from build123d import *

# Parameters (mm, degrees)
SKETCH1_W                      = 124
SKETCH1_H                      = 219.6
SKETCH1_R                      = 3.5
BOSS_EXTRUDE1_DEPTH            = 3.125
SKETCH2_R                      = 2.5
CUT_EXTRUDE1_DEPTH             = 10
M5_CLEARANCE_HOLE1_D           = 5.5
M5_CLEARANCE_HOLE1_DEPTH       = 10.1
M5_CLEARANCE_HOLE1_CSINK_D     = 5.55
M5_CLEARANCE_HOLE1_CSINK_ANGLE = 90
M5_CLEARANCE_HOLE1_TIP         = 1.652366702
M5_CLEARANCE_HOLE2_D           = 5.5
M5_CLEARANCE_HOLE2_DEPTH       = 10.1
M5_CLEARANCE_HOLE2_CSINK_D     = 5.55
M5_CLEARANCE_HOLE2_CSINK_ANGLE = 90
M5_CLEARANCE_HOLE2_TIP         = 1.652366702
M5_CLEARANCE_HOLE3_D           = 5.5
M5_CLEARANCE_HOLE3_CSINK_D     = 5.55
M5_CLEARANCE_HOLE3_CSINK_ANGLE = 90


with BuildPart() as part:
    # Sketch1 → Boss-Extrude1 (new body)
    with BuildSketch(Plane(origin=(0, 0, 0), x_dir=(1, 0, 0), z_dir=(0, 1, 0))):
        with Locations((62, 109.8)):
            Rectangle(SKETCH1_W, SKETCH1_H)
        with Locations((30, 71)):
            Circle(SKETCH1_R, mode=Mode.SUBTRACT)
    extrude(amount=BOSS_EXTRUDE1_DEPTH)

    # Sketch2 → Cut-Extrude1 (cut)
    with BuildSketch(Plane(origin=(0, 3.125, 0), x_dir=(1, 0, 0), z_dir=(0, 1, 0))):
        with Locations((10.312672757, 51)):
            Circle(SKETCH2_R)
        with Locations((50, 51)):
            Circle(SKETCH2_R)
        with Locations((50, 91)):
            Circle(SKETCH2_R)
        with Locations((10, 91)):
            Circle(SKETCH2_R)
    extrude(amount=-CUT_EXTRUDE1_DEPTH, mode=Mode.SUBTRACT)

    # M5 Clearance Hole1
    with Locations(Plane(origin=(0, 3.125, 0), x_dir=(1, 0, 0), z_dir=(0, 1, 0))):
        with Locations((24.25, 86), (35.75, 86), (35.75, 56), (24.25, 56)):
            CounterSinkHole(M5_CLEARANCE_HOLE1_D / 2, M5_CLEARANCE_HOLE1_CSINK_D / 2, depth=M5_CLEARANCE_HOLE1_DEPTH, counter_sink_angle=M5_CLEARANCE_HOLE1_CSINK_ANGLE)
            with Locations((0, 0, -(M5_CLEARANCE_HOLE1_DEPTH + M5_CLEARANCE_HOLE1_TIP / 2))):  # 118° drill point
                Cone(0, M5_CLEARANCE_HOLE1_D / 2, M5_CLEARANCE_HOLE1_TIP, mode=Mode.SUBTRACT)

    # M5 Clearance Hole2
    with Locations(Plane(origin=(0, 3.125, 0), x_dir=(1, 0, 0), z_dir=(0, 1, 0))):
        with Locations((22.049589497, 199.6), (72.049589497, 199.6), (104, 159.6), (104, 69.6)):
            CounterSinkHole(M5_CLEARANCE_HOLE2_D / 2, M5_CLEARANCE_HOLE2_CSINK_D / 2, depth=M5_CLEARANCE_HOLE2_DEPTH, counter_sink_angle=M5_CLEARANCE_HOLE2_CSINK_ANGLE)
            with Locations((0, 0, -(M5_CLEARANCE_HOLE2_DEPTH + M5_CLEARANCE_HOLE2_TIP / 2))):  # 118° drill point
                Cone(0, M5_CLEARANCE_HOLE2_D / 2, M5_CLEARANCE_HOLE2_TIP, mode=Mode.SUBTRACT)

    # M5 Clearance Hole3 (through all)
    with Locations(Plane(origin=(0, 3.125, 0), x_dir=(1, 0, 0), z_dir=(0, 1, 0))):
        with Locations((24, 124), (64, 124), (24, 18), (64, 18)):
            CounterSinkHole(M5_CLEARANCE_HOLE3_D / 2, M5_CLEARANCE_HOLE3_CSINK_D / 2, counter_sink_angle=M5_CLEARANCE_HOLE3_CSINK_ANGLE)


solid = part.part
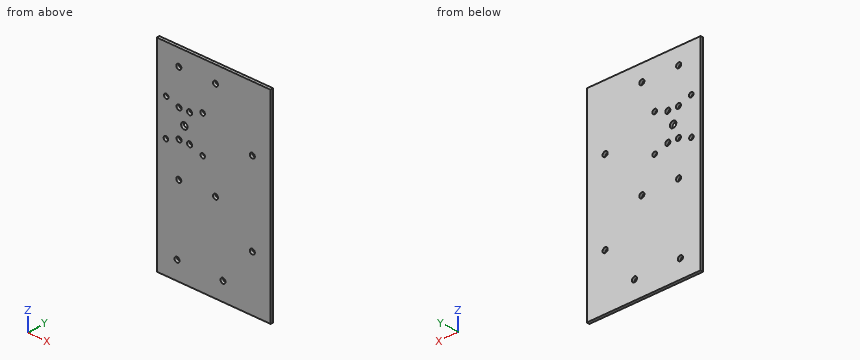
Could you check a few things on this model? Use its own coordinates, in mm. Round coordinates to 2 decimals unless told otherwise and drop trailing zeros. Write each loop counter-clockwise with the first axis right and the second up, starting at its lowest first coordinate (ties: lowest second). Pieces come first, ordered by that corner, then holes. Notation, with made-up numbers: (-37, -0.5) - (-27, -0.5) arc R22 cw to (-27, 6.5) - close; hole circle Ø2 at (45, 87.5). An arc over 180 degrees is marked (long way). Use a Markdown table: item, result.
Q1. I want a section at C-C (z = -91). List the corners of the cut face in (x, y) for me (3 decimals).
Output values:
| item | result |
|---|---|
| outline | (0, 0) - (7.5, 0) - (7.5, 3.125) - (0, 3.125) - close; (12.5, 0) - (47.5, 0) - (47.5, 3.125) - (12.5, 3.125) - close; (52.5, 0) - (124, 0) - (124, 3.125) - (52.5, 3.125) - close |
Q2. I want a section at A-A (x = 64). List the corners of the cut face in (y, z) for me (3 decimals).
Output values:
| item | result |
|---|---|
| outline | (0, -219.6) - (3.125, -219.6) - (3.125, -126.775) - (3.1, -126.75) - (0, -126.75) - close; (0, -121.25) - (3.1, -121.25) - (3.125, -121.225) - (3.125, -20.775) - (3.1, -20.75) - (0, -20.75) - close; (0, -15.25) - (3.1, -15.25) - (3.125, -15.225) - (3.125, 0) - (0, 0) - close |
Q3. Please list where these lines run through material, in increasing order: L1, parallel to Z at x = 50, y = 1.05; L2, parallel to Z at x = 35.75, y = 1.25; L3, parallel to X at y = 1.1, z = -18.
Output values:
| item | result |
|---|---|
| L1 | -219.6 to -93.5, -88.5 to -53.5, -48.5 to 0 |
| L2 | -219.6 to -88.75, -83.25 to -58.75, -53.25 to 0 |
| L3 | 0 to 21.25, 26.75 to 61.25, 66.75 to 124 |
Q4. For pin 1 (5 mm diameter, centred on x = 22.05, z = -199.6, fed in from +Y), with a flat end and sliding along its axis, tell me the tip position at first contact or that it passes through.
Output values:
| item | result |
|---|---|
| pin 1 | through |
Q5. I want a section at B-B (z = -199.6). List the corners of the cut face in (x, y) for me (3 decimals), plus the area to 3 significant figures.
Output values:
| item | result |
|---|---|
| outline | (0, 0) - (19.3, 0) - (19.3, 3.1) - (19.275, 3.125) - (0, 3.125) - close; (24.8, 0) - (69.3, 0) - (69.3, 3.1) - (69.275, 3.125) - (24.825, 3.125) - (24.8, 3.1) - close; (74.8, 0) - (124, 0) - (124, 3.125) - (74.825, 3.125) - (74.8, 3.1) - close |
| area | 353 mm2 |
